Solid Edge part; units mm, degrees
sketch "Sketch1" plane through (0, 0, 0) normal (0, 0, 1) x (1, 0, 0)
  line L0 (0, 0) -> (15.8, 0)
  line L1 (15.8, 0) -> (15.8, 7.8)
  line L2 (15.8, 7.8) -> (0, 7.8)
  line L3 (0, 7.8) -> (0, 0)
extrude "Protrusion1" add sketch "Sketch1" along normal blind 3.2
sketch "Sketch2" plane through (7.9, 3.9, 3.2) normal (0, 0, 1) x (1, 0, 0)
  circle A0 centre (4, 0) radius 2.4
  dimension "D1" = 4
extrude "ExtrudedProtrusion_2" add sketch "Sketch2" along normal blind 1.8
mirror "Mirror1" about plane through (7.9, 0, 0) normal (1, 0, 0) of "ExtrudedProtrusion_2"
sketch "Sketch3" plane through (7.9, 3.9, 0) normal (0, 0, -1) x (1, 0, 0)
  line L0 (-6.5, -2.5) -> (6.5, -2.5)
  line L1 (6.5, -2.5) -> (6.5, 2.5)
  line L2 (6.5, 2.5) -> (-6.5, 2.5)
  line L3 (-6.5, 2.5) -> (-6.5, -2.5)
extrude "ExtrudedCutout_1" cut sketch "Sketch3" against normal blind 2
sketch "Sketch4" plane through (7.9, 3.9, 2) normal (0, 0, -1) x (1, 0, 0)
  circle A0 centre (0, 0) radius 1.4
extrude "ExtrudedProtrusion_3" add sketch "Sketch4" along normal blind 2
sketch "Sketch5" plane through (7.9, 3.9, 2) normal (0, 0, -1) x (1, 0, 0)
  circle A0 centre (0, 0) radius 0.8
extrude "ExtrudedCutout_2" cut sketch "Sketch5" along normal blind 20
sketch "Sketch6" plane through (15.8, 3.9, 1.6) normal (1, 0, 0) x (0, 1, 0)
  line L0 (3.9, 3.3) -> (7.2, 14.4339)
  line L1 (7.2, 14.4339) -> (8.9, 14)
  line L2 (5.5, -1.6) -> (8.9, 14)
  line L3 (3.9, -1.6) -> (5.5, -1.6)
  line L4 (3.9, 3.3) -> (3.9, -1.6)
extrude "ExtrudedProtrusion_4" add sketch "Sketch6" against normal blind 1.5
sketch "Sketch7" plane through (15.8, 6.4, 8.0169) normal (1, 0, 0) x (0, 1, 0)
  line L0 (3, -8.0169) -> (3, -4.8169)
  line L1 (3, -4.8169) -> (1.4, -4.8169)
  line L2 (1.4, -4.8169) -> (1.4, -8.0169)
  line L3 (1.4, -8.0169) -> (3, -8.0169)
extrude "ExtrudedProtrusion_5" add sketch "Sketch7" against normal blind 15.8
sketch "Sketch8" plane through (14.3, 10.3, 8.0169) normal (-1, 0, 0) x (0, -0.2129497, -0.9770632)
  line L0 (4.8981, -0.1464) -> (-7.9415, -0.8278)
  line L1 (-7.9415, -0.8278) -> (-8.0034, 0.9256)
  line L2 (-8.0034, 0.9256) -> (3.5778, 1.7789)
  line L3 (3.5778, 1.7789) -> (5.2388, 1.4169)
  line L4 (5.2388, 1.4169) -> (4.8981, -0.1464)
extrude "ExtrudedProtrusion_6" add sketch "Sketch8" along normal blind 7.9
sketch "Sketch9" plane through (15.8, 6.4, 8.0169) normal (1, 0, 0) x (0, 0.2129497, 0.9770632)
  line L0 (-1.1517, -2.1492) -> (-0.6837, -4.2964)
  line L1 (-0.6837, -4.2964) -> (8.772, -4.6384)
  line L2 (8.772, -4.6384) -> (8.8339, -2.885)
  line L3 (8.8339, -2.885) -> (-1.1517, -2.1492)
extrude "Protrusion2" add sketch "Sketch9" along normal blind 7.7
sketch "Sketch10" plane through (19.65, 11.6261, 11.017) normal (0, 0.9687267, -0.2481301) x (0, -0.2481301, -0.9687267)
  line L0 (-4.7309, -3.85) -> (-4.7309, -2.85)
  line L1 (-4.7309, -2.85) -> (5.2762, -3.85)
  line L2 (5.2762, -3.85) -> (-4.7309, -3.85)
extrude "ExtrudedCutout_6" cut sketch "Sketch10" along normal mid plane 40
fillet "Round_2" radius 1 1 edges at (22.5001, 11.95, 15.8169)
fillet "Round_3" radius 0.2 1 edges at (23.4728, 9.3535, 6.434)
mirror "Mirror2" about plane through (7.9, 0, 0) normal (1, 0, 0) of "Protrusion2", "Round_2", "ExtrudedCutout_6", "ExtrudedProtrusion_4", "ExtrudedProtrusion_6", "Round_3"
sketch "Sketch11" plane through (15.8, 6.4, 7.8) normal (1, 0, 0) x (0, 1, 0)
  line L0 (4.6631, 1.0189) -> (2.5615, 1.0189)
  line L1 (2.5615, 1.0189) -> (1.8547, -1.366)
  line L2 (1.8547, -1.366) -> (4.0522, -1.366)
  line L3 (4.0522, -1.366) -> (4.6631, 1.0189)
extrude "ExtrudedCutout_7" cut sketch "Sketch11" along normal blind 20
mirror "Mirror3" about plane through (7.9, 0, 0) normal (1, 0, 0) of "ExtrudedCutout_7"
sketch "Sketch12" plane through (7.9, 4.7, 0) normal (0, 0, -1) x (1, 0, 0)
  line L0 (6.5, -3.5) -> (6.5, -1.7)
  line L1 (6.5, -1.7) -> (-6.5, -1.7)
  line L2 (-6.5, -1.7) -> (-6.5, -3.5)
  line L3 (-6.5, -3.5) -> (6.5, -3.5)
extrude "ExtrudedCutout_9" cut sketch "Sketch12" against normal blind 2
sketch "Sketch13" plane through (7.9, 4.8, 2) normal (0, 0, -1) x (1, 0, 0)
  line L0 (3.5, -3.4) -> (4.7, -3.4)
  line L1 (4.7, -3.4) -> (4.7, -1.8)
  line L2 (4.7, -1.8) -> (3.5, -1.8)
  line L3 (3.5, -1.8) -> (3.5, -3.4)
extrude "ExtrudedProtrusion_9" add sketch "Sketch13" along normal blind 1.9
mirror "Mirror4" about plane through (7.9, 0, 0) normal (1, 0, 0) of "ExtrudedProtrusion_9"
fillet "Round_4" radius 0.5 2 edges at (0, 10.0123, 8.8189) (15.8, 10.0123, 8.8189)
Can you work these out from the model? Positions are in its coordinate system, mm. A direction names the side the tool comes from. Coordinates: 2 decimals unless noted, no trailing zeros. Loops run counter-clockwise (first coordinate to the right, second up) from the corner with the lowest first, then second, coordinate; pieces in that order, holes last. Notation, with made-up numbers: (-20, 1) -> (39, 1) arc R22 ccw to (39, 29) -> close; hole circle Ø11 at (64.25, 37). An arc over 180 degrees is marked (long way). Put each result on its own line as item: value. Start each with the question number.
Q1. I want a section at C-C (z = 9.5). Write out the boundary of the cut face in (x, y).
Q2. For faces 4 (the face through (4, 7, 0.1)), 5 (the face through (-4, 10, 8.819)), 6 (the face through (19.448, 11.854, 11.908)), 7 (the face through (2.79, 1.77, 4.09)), which set-ups out of +Z, -Z, +X, -X, +Y, -Y let a thin tool reach every point of the face, with its end or its side?
Q3. I want a section at B-B (y = 6). Write out the boundary of the cut face in (x, z).
Q4. I'm going to push flat-ended pins straight in: P1, Ø1.3, axis at y = 7, z = 1, coming from the +X side; P2, Ø2.5, axis at x = -2.5, y = 10, coming from the -Z side; P3, Ø5, axis at x = 10.5, z = 4.5, coming from the +Y side; P4, Ø6, axis at y = 8.5, z = 7.5, coming from the -X side. Where does each tip first touch, or does it pass through?
Q5. I want a section at D-D (x = 4). Write out the boundary of the cut face in (y, z), plus the area to 3 significant figures.
Q6. Thinking about a two-plate mould opening in X: for faces 1 (the face through (-6.474, 11.88, 15.561)), 2 (the face through (15.061, 11.076, 7.691)), 3 (the face through (1.5, 10.6, 6.6)), which applies, pulls with the +X half, pulls with the -X half, needs draft (parallel to the pull), parting line crosses it, or undercut?
Q7. I want a section at A-A (x = 15). Write out the boundary of the cut face in (y, z).
Q8. If I drill on line 1 (X direction, y = 3.9, z = 0.8); line 2 (Y direction, x = 7.9, z = 0.55); line 3 (Z direction, x = 4, y = 5), over which ranges is the centre line in solid material (lowest first)? Write a range as [from, to].
Taken from the geometry:
1. outline: (-7.38, 9.16) -> (1.5, 9.16) -> (15.8, 9.16) -> (23.18, 9.16) -> (23.13, 11.24) -> (15.8, 11.24) -> (15.8, 11.47) -> (14.3, 11.47) -> (14.3, 11.13) -> (1.5, 11.13) -> (1.5, 11.47) -> (0, 11.47) -> (0, 11.24) -> (-7.33, 11.24) -> close
2. face 4: -Z
2. face 5: -Z, -X, +Y, -Y
2. face 6: -Z, +X, +Y
2. face 7: +Z
3. outline: (0, 0) -> (1.4, 0) -> (1.4, 2) -> (14.4, 2) -> (14.4, 0) -> (15.8, 0) -> (15.8, 3.2) -> (13.06, 3.2) -> (13.06, 5) -> (10.74, 5) -> (10.74, 3.2) -> (5.06, 3.2) -> (5.06, 5) -> (2.74, 5) -> (2.74, 3.2) -> (0, 3.2) -> close
4. P1: stops at x = 15.8
4. P2: stops at z = 8.82
4. P3: stops at y = 10.44
4. P4: stops at x = -7.45
5. outline: (0, 0) -> (1.4, 0) -> (1.4, 2) -> (6.6, 2) -> (6.6, 0.1) -> (8.2, 0.1) -> (8.2, 0) -> (9.4, 0) -> (9.4, 3.2) -> (12.8, 15.6) -> (11.1, 16.03) -> (7.8, 4.9) -> (7.8, 3.2) -> (6.3, 3.2) -> (6.3, 5) -> (1.5, 5) -> (1.5, 3.2) -> (0, 3.2) -> close
5. area: 52.5 mm2
6. face 1: pulls with the -X half
6. face 2: needs draft
6. face 3: undercut
7. outline: (0, 0) -> (9.4, 0) -> (12.8, 15.6) -> (11.1, 16.03) -> (7.8, 4.9) -> (7.8, 3.2) -> (0, 3.2) -> close
8. line 1: x = [0, 1.4], [6.5, 7.1], [8.7, 9.3], [14.4, 15.8]
8. line 2: y = [0, 1.4], [2.5, 3.1], [4.7, 5.3], [8.2, 9.4]
8. line 3: z = [2, 5]
